Study the drawing (mm; zero at the part's minimum x, y, z) and answer. A direction names the side the tool comes from. Give positions to 0.01 mm unless a question says otherwise; leave off trailing zeros. Loops run counter-clockwise (first coordinate to the right, second up) from the corner with the lowest first, then second, coordinate; pieces in that order, holes last. Notation, with made-up numbers: M 31.25,20 L 73.25,20 A6 cw 73.25,31 Z; hole C 36.25,-14 d7. An arc over 180 degrees is marked long. Return JSON: item names as keys, results as strings.
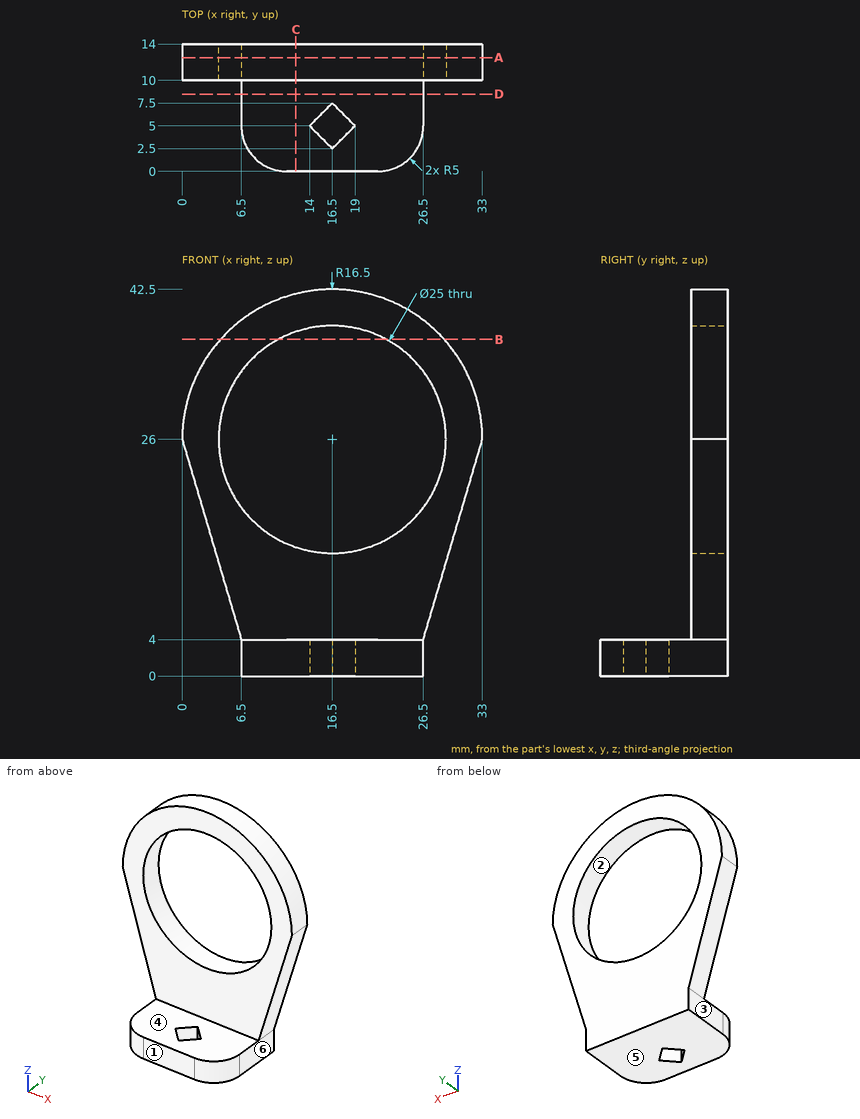
(1) Determine the mould class of the marked faces 1, 2 and 3 for opening direction X: released by +X, released by -X, zero draft, split by the parting line, or undercut.
Values follow:
{"face 1": "zero draft", "face 2": "undercut", "face 3": "released by -X"}
(2) Given pin 1 (4.5 mm diameter, centred on y = 9.5, z = 2, fed in from +X); pin 2 (5 mm diameter, centred on y = 11.5, z = 16, fed in from -X); pin 3 (3 mm diameter, centred on x = 19, y = 11, fed in from +Z), each flat-ended and moving along its own axis, determine where each tip first touches the part or whether it passes through.
Values follow:
{"pin 1": "x = 26.56", "pin 2": "x = 2.22", "pin 3": "z = 42.47"}
(3) The part is cut by section D-D (y = 8.5). Determine the outline of the cut face in (x, z), and give its area (3 significant figures).
Values follow:
{"outline": "M 6.5,0 L 26.5,0 L 26.5,4 L 6.5,4 Z", "area": "80.0 mm²"}
(4) The part is cut by section C-C (x = 12.5). Determine the outline of the cut face in (y, z).
Values follow:
{"outline": "M 0,0 L 14,0 L 14,14.16 L 10,14.16 L 10,4 L 0,4 Z; M 10,37.84 L 14,37.84 L 14,42.01 L 10,42.01 Z"}
(5) The part is cut by section A-A (y = 12.5). Determine the outline of the cut face in (x, z), and give its area (3 significant figures).
Values follow:
{"outline": "M 0,26 L 6.5,4 L 6.5,0 L 26.5,0 L 26.5,4 L 33,26 A16.5 ccw Z; hole C 16.5,26 d25", "area": "600 mm²"}
(6) Straight lines are drawn through the part: line 1 along Z through (x, y) = (16.5, 12.75); line 2 along Z through (x, y) = (21, 1); line 3 along Y through (x, z) = (11.5, 10.5). For each, find the intervals that lie inside material, in ascending order.
Values follow:
{"line 1": "0 to 13.5, 38.5 to 42.5", "line 2": "0 to 4", "line 3": "10 to 14"}
(7) The part is cut by section B-B (z = 37). Determine the outline of the cut face in (x, y), and give its area (3 significant figures).
Values follow:
{"outline": "M 4.2,10 L 10.56,10 L 10.56,14 L 4.2,14 Z; M 22.44,10 L 28.8,10 L 28.8,14 L 22.44,14 Z", "area": "50.9 mm²"}
(8) A tool of negligible diameter and unlimited length cuts with its end or side. For the marked faces 4, 5 and 6, from which of +Z, -Z, +X, -X, +Y, -Y can it reach the whole face along a straight path? Write none if from no direction.
Values follow:
{"face 4": "+Z, +X, -X, -Y", "face 5": "-Z, +X, -X, +Y, -Y", "face 6": "-Z, +X, +Y, -Y"}
